Verification items for the finished model (mm, model axes). Give positions to 0.01 mm unless a question says otherwise; leave off trailing zeros. Write each loop counter-clockwise with the first axis right and the second up, starting at its lowest first coordinate (ties: lowest second). Pieces come first, ordered by that corner, then holes. Notation, with made-up numbers: (34.5, 51) -> (62.5, 51) arc R20 ccw to (62.5, 58) -> close; hole circle Ø8 at (-27, 14). An arc over 180 degrees is marked (long way). Use CSV: the item, a comma, the result in double quotes. Start each with the question number.
```python
from build123d import *

# Parameters (mm, degrees)
F1_DEPTH = 3.175
F3_D     = 6.35
F4_D     = 6.35


with BuildPart() as f1:
    # F0 (on Front) → F1 (new body)
    with BuildSketch(Plane.XZ):
        Polygon((-157.175134, 323.548309), (-157.175134, -57.451691), (46.024866, -57.451691), (46.024866, 374.348309), (-90.500134, 374.348309), (-90.500134, 323.548309), align=None)
    extrude(amount=F1_DEPTH)

    # F3 (through all)
    with Locations(Plane.XZ.offset(3.175)):
        with Locations((-141.300134, -6.651691)):
            Hole(F3_D / 2)

    # F4 (through all)
    with Locations(Plane.XZ.offset(3.175)):
        with Locations((-141.300134, 133.048309), (-141.300134, 272.748309)):
            Hole(F4_D / 2)


solid = f1.part
```
(1) Section check A-A on y = -1.15. Record the cut outline in (x, z) (3 decimals).
(2) Go/stop test with flat-tipped pins: pin 1 (8.5 mm diameter, centred on x = -141.3, z = 133.05, fed in from -Y) (3 decimals); pin 2 (1.6 mm diameter, centred on x = -136, y = -2, fed in from +Z). Record where each tip stops, or that it passes through.
(3) Thickness scan on line 1 (X direction, y = -0.4, z = 272.5); line 2 (X direction, y = -0.9, z = 329); line 3 (Z direction, x = -134, y = -0.45). Record the ranges inside material, lowest first. Write a range as from..to.
Data:
1,outline,"(-157.175, -57.452) -> (46.025, -57.452) -> (46.025, 374.348) -> (-90.5, 374.348) -> (-90.5, 323.548) -> (-157.175, 323.548) -> close; hole circle Ø6.35 at (-141.3, -6.652); hole circle Ø6.35 at (-141.3, 133.048); hole circle Ø6.35 at (-141.3, 272.748)"
2,pin 1,"stops at y = -3.175"
2,pin 2,"stops at z = 323.55"
3,line 1,"x = -157.18..-144.47, -138.13..46.02"
3,line 2,"x = -90.5..46.02"
3,line 3,"z = -57.45..323.55"
